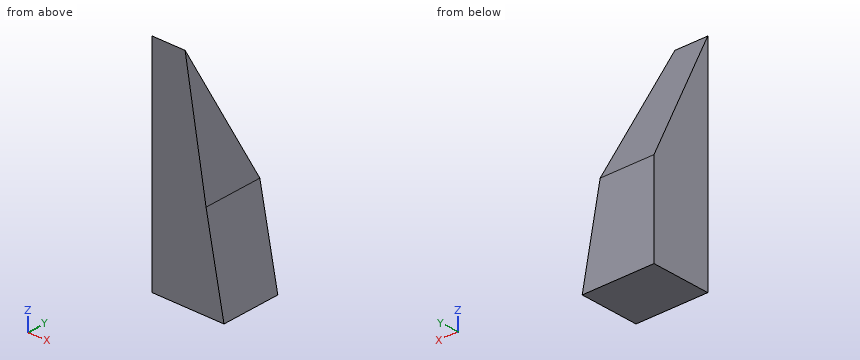
from build123d import *

# Parameters (mm, degrees)
BOSS_EXTRUDE1_DEPTH = 508
CUT_EXTRUDE1_DEPTH  = 508
BOSS_EXTRUDE2_DEPTH = 508


with BuildPart() as part:
    # Sketch1 → Boss-Extrude1 (new body)
    with BuildSketch(Plane(origin=(0, 0, 0), x_dir=(1, 0, 0), z_dir=(0, 1, 0))):
        Polygon((0, 1066.8), (0, 0), (279.4, 0), (457.2, 1066.8), align=None)
    extrude(amount=BOSS_EXTRUDE1_DEPTH)

    # Sketch2 → Cut-Extrude1 (cut)
    with BuildSketch(Plane.ZY):
        Polygon((0, 0), (-1066.8, 508), (-1066.8, 732.672417782), (0, 732.672417782), align=None)
    extrude(amount=-CUT_EXTRUDE1_DEPTH, mode=Mode.SUBTRACT)

    # Sketch3 → Boss-Extrude2 (add)
    with BuildSketch(Plane.XZ):
        Polygon((0, -1066.8), (0, -1854.2), (609.6, -1854.2), (457.2, -1066.8), align=None)
    extrude(amount=-BOSS_EXTRUDE2_DEPTH)


solid = part.part
The model under review builds one solid part; all positions refer to its coordinate system, in mm. Round coordinates to 2 decimals unless told otherwise and drop trailing zeros. Loops run counter-clockwise (first coordinate to the right, second up) from the corner with the lowest first, then second, coordinate; pieces in that order, holes last. Notation, with made-up numbers: (13.25, 1.5) -> (38.25, 1.5) arc R21 ccw to (38.25, 32.5) -> close; hole circle Ø3 at (-32.5, 87). An arc over 180 degrees is marked (long way). Write item = value, one per line. Start each with the question number.
Item 1: Take a section at A-A on y = 161. Give the boundary of the cut face in (x, z), plus the area to 3 significant figures.
Item 2: Take a section at C-C on z = -409.5. Give the boundary of the cut face in (x, y), plus the area to 3 significant figures.
Item 3: Take a section at D-D on y = 399.5. Give the boundary of the cut face in (x, z) (3 decimals).
Item 4: Insertion check: pin 1 (3 mm diameter, centred on x = 330.5, y = 383.5, fed in from +Z); pin 2 (6 mm diameter, centred on y = 334, z = -818.5, fed in from +X); pin 3 (1 mm diameter, centred on x = 321, y = 396, fed in from +Z). Each pin has a flat end and moves straight along its axis. Give the tip position at first contact, or say it passes through.
Item 5: Take a section at B-B on x = 480. Give the boundary of the cut face in (y, z).
Item 6: To check wall thickness, follow L1, parallel to Y at x = 273, z = -1026; L2, parallel to Z at x = 146, y = 400; L3, parallel to X at y = 396, z = -1772. State the ranges of each line that lie inside material, in increasing order.
Result:
q1.outline = (0, -1854.2) -> (609.6, -1854.2) -> (457.2, -1066.8) -> (335.75, -338.1) -> (0, -338.1) -> close
q1.area = 709,000 mm²
q2.outline = (0, 0) -> (347.65, 0) -> (347.65, 195) -> (0, 195) -> close
q2.area = 67,800 mm²
q3.outline = (0, -1854.2) -> (609.6, -1854.2) -> (457.2, -1066.8) -> (419.225, -838.95) -> (0, -838.95) -> close
q4.pin_1 = -802.2
q4.pin_2 = 416.32
q4.pin_3 = -830.55
q5.outline = (0, -1854.2) -> (508, -1854.2) -> (508, -1184.6) -> (0, -1184.6) -> close
q6.L1 = 0 to 488.57
q6.L2 = -1854.2 to -840
q6.L3 = 0 to 593.69
